```python
from build123d import *

# Parameters (mm, degrees)
SKETCH1_W           = 120
SKETCH1_H           = 120
BOSS_EXTRUDE1_DEPTH = 1.5
SKETCH4_R           = 2.5
CUT_EXTRUDE2_DEPTH  = 1.5
SKETCH7_R           = 1.5
CUT_EXTRUDE3_DEPTH  = 1.5
SKETCH8_W           = 94
SKETCH8_H           = 106
CUT_EXTRUDE4_DEPTH  = 1.5
FILLET1_R           = 0.5


with BuildPart() as part:
    # Sketch1 → Boss-Extrude1 (new body)
    with BuildSketch(Plane(origin=(0, 0, 0), x_dir=(1, 0, 0), z_dir=(0, 1, 0))):
        Rectangle(SKETCH1_W, SKETCH1_H)
    extrude(amount=BOSS_EXTRUDE1_DEPTH)

    # Sketch4 → Cut-Extrude2 (cut)
    with BuildSketch(Plane(origin=(0, 0, 0), x_dir=(1, 0, 0), z_dir=(0, 1, 0))):
        with Locations((-22.5, 0)):
            Circle(SKETCH4_R)
        with Locations((22.5, 0)):
            Circle(SKETCH4_R)
    extrude(amount=CUT_EXTRUDE2_DEPTH, mode=Mode.SUBTRACT)

    # Sketch7 → Cut-Extrude3 (cut)
    with BuildSketch(Plane(origin=(0, 0, 0), x_dir=(1, 0, 0), z_dir=(0, 1, 0))):
        with Locations((-53, 53)):
            Circle(SKETCH7_R)
        with Locations((53, 53)):
            Circle(SKETCH7_R)
        with Locations((-53, -53)):
            Circle(SKETCH7_R)
        with Locations((53, -53)):
            Circle(SKETCH7_R)
    extrude(amount=CUT_EXTRUDE3_DEPTH, mode=Mode.SUBTRACT)

    # Sketch8 → Cut-Extrude4 (cut)
    with BuildSketch(Plane(origin=(0, 0, 0), x_dir=(1, 0, 0), z_dir=(0, 1, 0))):
        Rectangle(SKETCH8_W, SKETCH8_H)
    extrude(amount=CUT_EXTRUDE4_DEPTH, mode=Mode.SUBTRACT)

    # Fillet1
    fillet1_edges = [part.edges().sort_by_distance(p)[0] for p in [
        (0, 1.5, -53),
        (47, 0.75, -53),
        (0, 0, -53),
        (47, 1.5, 0),
        (47, 0, 0),
        (0, 1.5, 53),
        (-47, 0.75, 53),
        (0, 0, 53),
        (-47, 1.5, 0),
        (-47, 0.75, -53),
        (-47, 0, 0),
    ]]
    fillet(fillet1_edges, radius=FILLET1_R)


solid = part.part
```
Design review of the part built by this model. Coordinates are the model's own, in mm. Give positions to 0.01 mm unless a question says otherwise; leave off trailing zeros. Loops run counter-clockwise (first coordinate to the right, second up) from the corner with the lowest first, then second, coordinate; pieces in that order, holes last. Notation, with made-up numbers: (-15.75, 75.5) -> (30.25, 75.5) arc R16 ccw to (30.25, 103.5) -> close; hole circle Ø11 at (55, -39). An arc over 180 degrees is marked (long way). One line per item, written item: value.
Q1. We need section B-B on z = 41. Give the boundary of the cut face in (x, y), and give its area (3 significant figures).
Numbers:
outline: (-60, 0) -> (-47.5, 0) arc R0.5 ccw to (-47, 0.5) -> (-47, 1) arc R0.5 ccw to (-47.5, 1.5) -> (-60, 1.5) -> close; (47, 0.5) arc R0.5 ccw to (47.5, 0) -> (60, 0) -> (60, 1.5) -> (47.5, 1.5) arc R0.5 ccw to (47, 1) -> close
area: 38.8 mm^2
Q2. For pin 1 Ø4 at (x, z) = (53, 53) entering from -Y, flat-tipped, find the tip position at first contact; note if it passes through.
Numbers:
pin 1: stops at y = 0
Q3. For L1, parallel to Z at x = 53, y = 1.2; L2, parallel to X at y = 0.5, z = -16; L3, parallel to Z at x = 18.5, y = 0.65, list the stretches that pass through material, from the lowest coordinate up.
Numbers:
L1: z = -60 to -54.5, -51.5 to 51.5, 54.5 to 60
L2: x = -60 to -47, 47 to 60
L3: z = -60 to -53, 53 to 60
Q4. Draft analysis for pull direction Z (two halves, no side actions). For faces 1 (the cylindrical face through (51.8, 0.7, 53.9)), 2 (the flat face through (4, 0, -54)), state which applies: pulls with the +Z half, pulls with the -Z half, needs draft (parallel to the pull), parting line crosses it, or undercut.
Numbers:
face 1: undercut
face 2: needs draft
Q5. We need section A-A on x = -21. Give the boundary of the cut face in (y, z).
Numbers:
outline: (0, -60) -> (1.5, -60) -> (1.5, -53.5) arc R0.5 ccw to (1, -53) -> (0.5, -53) arc R0.5 ccw to (0, -53.5) -> close; (0, 53.5) arc R0.5 ccw to (0.5, 53) -> (1, 53) arc R0.5 ccw to (1.5, 53.5) -> (1.5, 60) -> (0, 60) -> close
Q6. We need section C-C on x = -53. Give the boundary of the cut face in (y, z).
Numbers:
outline: (0, -60) -> (1.5, -60) -> (1.5, -54.5) -> (0, -54.5) -> close; (0, -51.5) -> (1.5, -51.5) -> (1.5, 51.5) -> (0, 51.5) -> close; (0, 54.5) -> (1.5, 54.5) -> (1.5, 60) -> (0, 60) -> close
